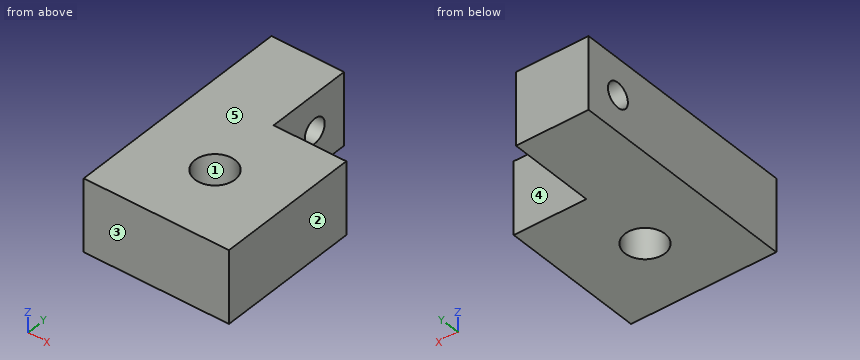
Autodesk Inventor part; units mm, degrees
ref_plane "YZ Plane" through (0, 0, 0) normal (1, 0, 0) x (0, 1, 0)
ref_plane "XZ Plane" through (0, 0, 0) normal (0, 1, 0) x (-1, 0, 0)
ref_plane "XY Plane" through (0, 0, 0) normal (0, 0, 1) x (1, 0, 0)
sketch "スケッチ4" plane through (0, 0, 0) normal (0, 0, 1) x (1, 0, 0)
  line L0 (0, 0) -> (20, 0)
  line L1 (20, 0) -> (20, 20)
  line L2 (0, 32) -> (0, 0)
  line L3 (0, 32) -> (10, 32)
  line L4 (10, 32) -> (10, 20)
  line L5 (10, 20) -> (20, 20)
  line L6 (10, 0) -> (10, 7.8024) construction
  circle A0 centre (10, 10) radius 2.75
  dimension "d19" = 20
  dimension "d20" = 32
  dimension "d21" = 12
  dimension "d22" = 10
  dimension "d24" = 5.5
  dimension "d25" = 10
extrude "押し出し4" add sketch "スケッチ4" along normal blind 10
sketch "スケッチ5" plane through (0, 0, 0) normal (-1, 0, 0) x (0, 0, 1)
  line L0 (0, 32) -> (10, 32)
  line L1 (5, 32) -> (5, 27) construction
  circle A0 centre (5, 27) radius 1.7
  point P0 (0, 0)
  dimension "d28" = 3.4
  dimension "d29" = 5
extrude "押し出し5" cut sketch "スケッチ5" against normal blind 10
properties part number "pixymount1"
Input: part model. Units: mm. Frame: model coordinates. Face numbers are marked on the shaded views. A direction names the side the tool comes from. Coordinates: 2 decimals unless noted, no trailing zeros. Loops run counter-clockwise (first coordinate to the right, second up) from the corner with the lowest first, then second, coordinate; pieces in that order, holes last. Notation, with made-up numbers: M 14.25,85.25 L 55.25,85.25 A7 cw 55.25,96.25 Z; hole C 61,0 d8. An arc over 180 degrees is marked long. Use a Markdown table: item, result. Add a question column.
1) Draft query along X for the marked faces 1, 2 and 3. Return one class per face: +X half, -X half, draft (parallel to the pull), parting line (faces both ways), or undercut.
2) Section B-B, the plane y = 10. Return the cut outline in (x, z), plus the area to 3 significant figures.
3) Section C-C, the plane x = 3.75. Return the cut outline in (y, z), plus the area to 3 significant figures.
4) Section A-A, the plane z = 5. Return the cut outline in (x, y).
5) Pin query (flat end, axial travel): P1, Ø1.5, axis at x = 12.5, z = 5, coming from the +Y side; P2, Ø5, axis at y = 28, z = 4, coming from the +X side. Return the tip coordinate at first contact, or that it passes through.
6) Section D-D, the plane y = 27. Return the cut outline in (x, z).
7) Line query: L1, parallel to Y at x = 5.75, z = 5; L2, parallel to X at y = 26, z = 3.25; L3, parallel to Y at x = 14.5, z = 7.5. Output: solid intervals per line, ascending. Write a range as from..to.
8) Set-up query: the marked faces 4 and 5. Return all of +Z, -Z, +X, -X, +Y, -Y with unobstructed straight access to the full face (end or side cutting, diameter ignored); none if empty.
Answer below:
| question | item | result |
|---|---|---|
| 1 | face 1 | undercut |
| 1 | face 2 | +X half |
| 1 | face 3 | draft |
| 2 | outline | M 0,0 L 7.25,0 L 7.25,10 L 0,10 Z; M 12.75,0 L 20,0 L 20,10 L 12.75,10 Z |
| 2 | area | 145 mm2 |
| 3 | outline | M 0,0 L 32,0 L 32,10 L 0,10 Z; hole C 27,5 d3.4 |
| 3 | area | 311 mm2 |
| 4 | outline | M 0,0 L 20,0 L 20,20 L 10,20 L 10,25.3 L 0,25.3 Z; M 0,28.7 L 10,28.7 L 10,32 L 0,32 Z; hole C 10,10 d5.5 |
| 5 | P1 | y = 20 |
| 5 | P2 | x = 10 |
| 6 | outline | M 0,0 L 10,0 L 10,3.3 L 0,3.3 Z; M 0,6.7 L 10,6.7 L 10,10 L 0,10 Z |
| 7 | L1 | 0..25.3, 28.7..32 |
| 7 | L2 | 0..10 |
| 7 | L3 | 0..20 |
| 8 | face 4 | +Z, -Z, +X, +Y |
| 8 | face 5 | +Z, +X, -X, +Y, -Y |
